Work out the finished part from the listing and answer in its coordinate system (mm). Face numbers are marked on the shaded views. A direction names the side the tool comes from. Round coordinates to 2 decimals unless told otherwise and drop trailing zeros. Write each loop counter-clockwise with the first axis right and the second up, starting at its lowest first coordinate (ties: lowest second). Pieces come first, ordered by that corner, then holes. Notation, with made-up numbers: (75.25, 58) -> (108.25, 58) arc R29 ccw to (108.25, 94) -> close; hole circle Ø6 at (83.25, -36). An arc over 180 degrees is marked (long way). One line per item, written item: value.
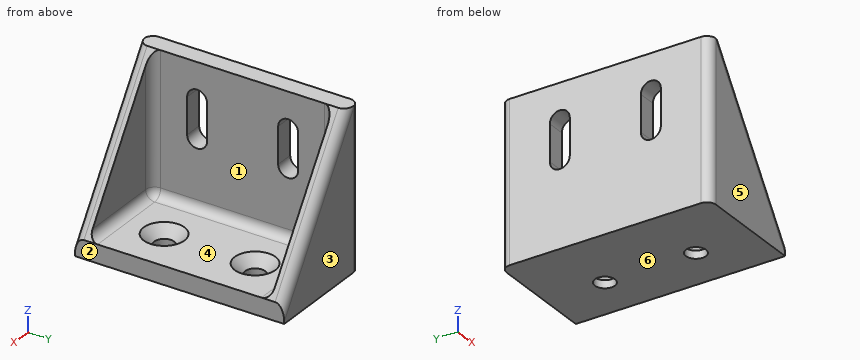
```python
from build123d import *

# Parameters (mm, degrees)
F1_DEPTH       = 40
F3_DEPTH       = 4
F5_D           = 4.4
F5_CSINK_D     = 8.96
F5_CSINK_ANGLE = 90
F7_DEPTH       = 3
F10_R          = 2
F11_T1_DEPTH   = 45


# Not quite as in the source:
# - a fillet or chamfer that OpenCascade refuses, or shapes differently, is made with other operations: its cross-section is extruded or revolved along the edge and cut away or added


with BuildPart() as f1:
    # F0 (on Front) → F1 (new body)
    with BuildSketch(Plane.XZ):
        Polygon((-12.4999986735, 17.5), (-12.4999986735, -17.5), (12.4999986735, -17.5), (12.4999986735, -13.5), (-8.4999986735, -13.5), (-8.4999986735, 17.5), align=None)
    extrude(amount=F1_DEPTH)

    # F2 (on face) → F3 (cut, through all)
    with BuildSketch(Plane.YZ.offset(-8.4999986735)):
        with BuildLine():
            ThreePointArc((-27.8069023984, 9.5), (-30, 11.6930976016), (-32.1930976016, 9.5))
            Line((-32.1930976016, 9.5), (-32.1930976016, 1.5))
            ThreePointArc((-32.1930976016, 1.5), (-30, -0.6930976016), (-27.8069023984, 1.5))
            Line((-27.8069023984, 1.5), (-27.8069023984, 9.5))
        make_face()
        with BuildLine():
            Line((-7.8069023984, 1.5), (-7.8069023984, 9.5))
            ThreePointArc((-7.8069023984, 9.5), (-10, 11.6930976016), (-12.1930976016, 9.5))
            Line((-12.1930976016, 9.5), (-12.1930976016, 1.5))
            ThreePointArc((-12.1930976016, 1.5), (-10, -0.6930976016), (-7.8069023984, 1.5))
        make_face()
    extrude(amount=-F3_DEPTH, mode=Mode.SUBTRACT)

    # F5 (through all)
    with Locations(Plane.XY.offset(-13.5)):
        with Locations((2.4999986735, -30), (2.4999986735, -10)):
            CounterSinkHole(F5_D / 2, F5_CSINK_D / 2, counter_sink_angle=F5_CSINK_ANGLE)

    # F6 (on face) → F7 (join)
    with BuildSketch(Plane.XZ.offset(40)):
        Polygon((12.4999986735, -13.5), (-8.4999986735, 17.5), (-12.4999986735, 17.5), (-12.4999986735, -17.5), (12.4999986735, -17.5), align=None)
    extrude(amount=F7_DEPTH)

    # F9: F1 across plane


with BuildPart() as f1_1:
    add(f1.part)
    add(f1.part.mirror(Plane(origin=(-5.812499541, -20, -5.812499541), x_dir=(1, 0, 0), z_dir=(0, 1, 0))))

    # F10
    f10_edges = [f1_1.edges().sort_by_distance(p)[0] for p in [
        (-8.499999, -40, 2),
        (2, -40, -13.5),
        (-8.499999, -20, -13.5),
        (2, 0, -13.5),
        (-8.499999, 0, 2),
        (2, 3, 2),
        (2, -43, 2),
    ]]
    fillet(f10_edges, radius=F10_R)

    # F11: fillet of radius 2 on 2 edges, made by hand

    # F11_s2 → F11_t1 (cut)
    with BuildSketch(Plane.XY.offset(-22.5)):
        with BuildLine():
            ThreePointArc((-10.4999986735, 3), (-11.9142122359, 2.4142135624), (-12.4999986735, 1))
            Line((-12.4999986735, 1), (-12.4999986735, 3))
            Line((-12.4999986735, 3), (-10.4999986735, 3))
        make_face()
        with BuildLine():
            ThreePointArc((-12.4999986735, -41), (-11.9142122359, -42.4142135624), (-10.4999986735, -43))
            Line((-10.4999986735, -43), (-12.4999986735, -43))
            Line((-12.4999986735, -43), (-12.4999986735, -41))
        make_face()
    extrude(amount=F11_T1_DEPTH, mode=Mode.SUBTRACT)


solid = f1_1.part
```
(1) For a pull along Y with two mould halves and no side action, classify the marked faces 3, 4, 5 and 6 as pulls with the +Y half, pulls with the -Y half, needs draft (parallel to the pull), parting line crosses it, or undercut.
Reported:
face 3: pulls with the +Y half
face 4: undercut
face 5: pulls with the -Y half
face 6: needs draft
(2) Consider probe 1 along Y at (x, z) = (-4.75, 7.5); probe 2 along X at (y, z) = (-10, -16); probe 3 along Z at (x, y) = (2, -16.5). Determine where each line is inside the solid, lowest interval first.
Reported:
probe 1: y = -43 to -40, 0 to 3
probe 2: x = -12.5 to 0.3, 4.7 to 12.5
probe 3: z = -17.5 to -13.5
(3) Find section C-C on x = 3.5. Give the number of separate pieces and of enclosed holes in the cut face, plus the area to 3 significant figures.
Reported:
separate pieces: 3
enclosed holes: 0
area: 220 mm2
(4) Flat-ended cylindrical pins translate along their axes: pin 1 Ø2.5 at (x, y) = (2.5, -10) entering from -Z; pin 2 Ø5 at (y, z) = (-15, -3) entering from +X; pin 3 Ø5 at (x, y) = (6, -9.5) entering from +Z; pin 4 Ø2 at (x, z) = (-11, 5.5) entering from +Y. Find the tip coordinate at first contact, or state that the pin passes through.
Reported:
pin 1: passes through
pin 2: stops at x = -8.5
pin 3: stops at z = -13.5
pin 4: stops at y = 3
(5) A tool of negligible diameter and unlimited length cuts with its end or side. For the marked faces 1 and 2, from which of +Z, -Z, +X, -X, +Y, -Y can it reach the whole face along a straight path? Write none if from no direction.
Reported:
face 1: +Z, +X
face 2: +Z, -Z, +X, +Y, -Y
(6) Find section B-B on y = -16. Give the vertices of the cut face in (x, z).
Reported:
outline: (-12.5, -17.5) -> (12.5, -17.5) -> (12.5, -13.5) -> (-6.5, -13.5) arc R2 cw to (-8.5, -11.5) -> (-8.5, 17.5) -> (-12.5, 17.5) -> close
(7) Find section A-A on y = -30. Give the vertices of the cut face in (x, z).
Reported:
outline: (-12.5, -17.5) -> (0.3, -17.5) -> (0.3, -15.78) -> (-1.98, -13.5) -> (-6.5, -13.5) arc R2 cw to (-8.5, -11.5) -> (-8.5, -0.69) -> (-12.5, -0.69) -> close; (-12.5, 11.69) -> (-8.5, 11.69) -> (-8.5, 17.5) -> (-12.5, 17.5) -> close; (4.7, -17.5) -> (12.5, -17.5) -> (12.5, -13.5) -> (6.98, -13.5) -> (4.7, -15.78) -> close
